```python
from build123d import *

# Parameters (mm, degrees)
BOSS_EXTRU_1_DEPTH           = 200
CHANFREIN1_SIZE              = 2
ESQUISSE2_R                  = 3
ENL_V_MAT_EXTRU_1_DEPTH      = 1
ENL_V_MAT_EXTRU_1_DEPTH_BACK = 26
CHANFREIN2_SIZE              = 2
CHANFREIN3_SIZE              = 2


with BuildPart() as part:
    # Esquisse1 → Boss.-Extru.1 (new body)
    with BuildSketch(Plane.XY):
        Polygon((-14, 10.714285714), (-14, -12.5), (14, -12.5), (14, 10.714285714), (15.100215679, 10.714285714), (15.100215679, 12.5), (14, 12.5), (10.899784321, 12.5), (10.899784321, 10.714285714), (12, 10.714285714), (12, -10.714285714), (-12, -10.714285714), (-12, 10.714285714), (-10.899784321, 10.714285714), (-10.899784321, 12.5), (-14, 12.5), (-15.100215679, 12.5), (-15.100215679, 10.714285714), align=None)
    extrude(amount=BOSS_EXTRU_1_DEPTH)

    # Chanfrein1
    chanfrein1_edges = [part.edges().sort_by_distance(p)[0] for p in [
        (14, -12.5, 100),
        (-14, -12.5, 100),
    ]]
    chamfer(chanfrein1_edges, length=CHANFREIN1_SIZE)

    # Esquisse2 → Enlèv. mat.-Extru.1 (cut, two sides)
    with BuildSketch(Plane.XZ.offset(12.5)) as enl_v_mat_extru_1_sk:
        with Locations((0, 100)):
            Circle(ESQUISSE2_R)
        with Locations((0, 175.000381003)):
            Circle(ESQUISSE2_R)
        with Locations((0, 24.999618997)):
            Circle(ESQUISSE2_R)
    extrude(amount=ENL_V_MAT_EXTRU_1_DEPTH, mode=Mode.SUBTRACT)
    extrude(enl_v_mat_extru_1_sk.sketch, amount=-ENL_V_MAT_EXTRU_1_DEPTH_BACK, mode=Mode.SUBTRACT)

    # Chanfrein2
    chanfrein2_edges = [part.edges().sort_by_distance(p)[0] for p in [
        (-12, -10.714285714, 100),
    ]]
    chamfer(chanfrein2_edges, length=CHANFREIN2_SIZE)

    # Chanfrein3
    chanfrein3_edges = [part.edges().sort_by_distance(p)[0] for p in [
        (12, -10.714285714, 100),
    ]]
    chamfer(chanfrein3_edges, length=CHANFREIN3_SIZE)


solid = part.part
```
Part model, mm, in its own coordinate system. A direction names the side the tool comes from. Coordinates: 2 decimals unless noted, no trailing zeros. Order: outer loops, then holes, each group sorted by start corner. A loop starts at its lowest first (then second) coordinate and runs counter-clockwise, first axis right, second up. Notation, with made-up numbers: (49.25, 5) -> (90.25, 5) arc R18 cw to (90.25, 11) -> close; hole circle Ø7 at (16.5, -31.75). An arc over 180 degrees is marked (long way). Put each result on its own line as item: value. Start each with the question number.
(1) Mould opens along Y. For faces 5 (the face through (12, 1, 99)), 6 (the face through (0, -11, 200)), 7 (the face through (13, 12.5, 99)), 8 (the face through (-12, 1, 99)) say: pulls with the +Y half, pulls with the -Y half, needs draft (parallel to the pull), parting line crosses it, or undercut.
(2) Band-saw the part on B-B (x = 0). Give the cut face in (y, z).
(3) Band-saw the part on D-D (z = 159). Give the cut face in (x, y).
(4) Band-saw the part on C-C (z = 100). Give the cut face in (x, y).
(5) Probe line 1 along Z through (x, y) = (0, -11.5); line 2 along X through (y, z) = (0.25, 64); line 3 along X through (y, z) = (11.25, 108). List the from-to ranges inside material, lowest first. Write a range as [from, to].
(6) Band-saw the part on A-A (y = -5.5). Give the cut face in (x, z).
(7) Which spindle directions (+Z, -Z, +X, -X, +Y, -Y) get a long thin tool onto all of the face, cutting with end or side? Do faces 1 (the face through (14, 0, 99)), 2 (the face through (0, -12, 28)), 3 (the face through (-4, -10.714, 99)), 4 (the face through (-14, 0, 99)). Say none if no direction does.
(8) Pin check, flat tips, straight feed: pin 1 Ø10 at (y, z) = (-0.5, 25) entering from +X; pin 2 Ø5 at (x, y) = (-11.5, 0.5) entering from -Z; pin 3 Ø1 at (y, z) = (-8, 101) entering from -X; pin 4 Ø5.5 at (x, z) = (0, 25) entering from +Y. Stop position of each tip, or through.
Determined:
1. face 5: undercut
1. face 6: needs draft
1. face 7: pulls with the +Y half
1. face 8: undercut
2. outline: (-12.5, 0) -> (-10.71, 0) -> (-10.71, 22) -> (-12.5, 22) -> close; (-12.5, 28) -> (-10.71, 28) -> (-10.71, 97) -> (-12.5, 97) -> close; (-12.5, 103) -> (-10.71, 103) -> (-10.71, 172) -> (-12.5, 172) -> close; (-12.5, 178) -> (-10.71, 178) -> (-10.71, 200) -> (-12.5, 200) -> close
3. outline: (-15.1, 10.71) -> (-14, 10.71) -> (-14, -10.5) -> (-12, -12.5) -> (12, -12.5) -> (14, -10.5) -> (14, 10.71) -> (15.1, 10.71) -> (15.1, 12.5) -> (10.9, 12.5) -> (10.9, 10.71) -> (12, 10.71) -> (12, -8.71) -> (10, -10.71) -> (-10, -10.71) -> (-12, -8.71) -> (-12, 10.71) -> (-10.9, 10.71) -> (-10.9, 12.5) -> (-15.1, 12.5) -> close
4. outline: (-15.1, 10.71) -> (-14, 10.71) -> (-14, -10.5) -> (-12, -12.5) -> (-3, -12.5) -> (-3, -10.71) -> (-10, -10.71) -> (-12, -8.71) -> (-12, 10.71) -> (-10.9, 10.71) -> (-10.9, 12.5) -> (-15.1, 12.5) -> close; (3, -12.5) -> (12, -12.5) -> (14, -10.5) -> (14, 10.71) -> (15.1, 10.71) -> (15.1, 12.5) -> (10.9, 12.5) -> (10.9, 10.71) -> (12, 10.71) -> (12, -8.71) -> (10, -10.71) -> (3, -10.71) -> close
5. line 1: z = [0, 22], [28, 97], [103, 172], [178, 200]
5. line 2: x = [-14, -12], [12, 14]
5. line 3: x = [-15.1, -10.9], [10.9, 15.1]
6. outline: (-14, 0) -> (-12, 0) -> (-12, 200) -> (-14, 200) -> close; (12, 0) -> (14, 0) -> (14, 200) -> (12, 200) -> close
7. face 1: +Z, -Z, +X, -Y
7. face 2: +Y, -Y
7. face 3: +Z, -Z, +Y
7. face 4: +Z, -Z, -X, -Y
8. pin 1: stops at x = 14
8. pin 2: stops at z = 0
8. pin 3: stops at x = -14
8. pin 4: passes through
